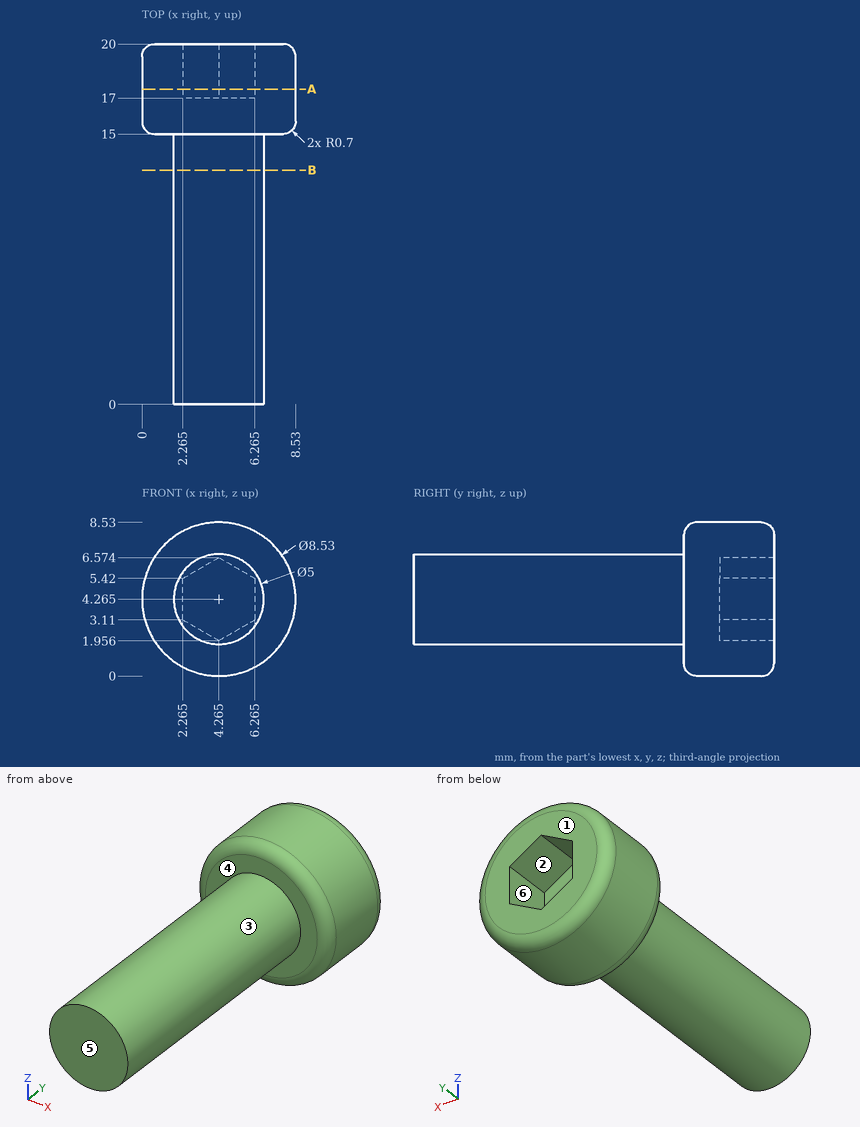
Design review of the part shown in the three views and the two pictorial views. Dimensions are in mm from the part's minimum x, y and z. A direction names the side the tool comes from. Round coordinates to 2 decimals unless told otherwise and drop trailing zeros. Loops run counter-clockwise (first coordinate to the right, second up) from the corner with the lowest first, then second, coordinate; pieces in that order, holes last. Notation, with made-up numbers: M -15.5,9 L 31.5,9 A27 ccw 31.5,26 Z; hole C -39.5,50 d2. An arc over 180 degrees is marked long. Put each result on its own line as item: value.
Q1. Mouldability with a two-part tool opening along X and no side actions: class the marked faces 1, 2 and 3 as released by +X, released by -X, zero draft, split by the parting line, or undercut.
Result set:
face 1: zero draft
face 2: undercut
face 3: split by the parting line
Q2. For pin 1 (4 mm diameter, centred on y = 12.5, z = 6.5, fed in from +X), flat-tipped, find the tip position at first contact; note if it passes through.
Result set:
pin 1: stops at x = 6.75
Q3. Consider section B-B, the plane y = 13. Give the boundary of the cut face in (x, z) (1 decimal).
Result set:
outline: C 4.3,4.3 d5
Q4. To check wall thickness, follow L1, parallel to Y at x = 2.5, z = 5.5; L2, parallel to Z at x = 0.5, y = 17 (1 decimal); L3, parallel to Y at x = 1.5, z = 5.5. State the ranges of each line that lie inside material, in increasing order.
Result set:
L1: y = 0 to 17
L2: z = 2.3 to 6.3
L3: y = 15 to 20
Q5. Consider section A-A, the plane y = 17.5. Give the boundary of the cut face in (x, z) (1 decimal).
Result set:
outline: C 4.3,4.3 d8.5; hole M 2.3,3.1 L 4.3,2 L 6.3,3.1 L 6.3,5.4 L 4.3,6.6 L 2.3,5.4 Z
Q6. Machinability: for the marked faces 4, 5 and 6, which of the approach directions +Z, -Z, +X, -X, +Y, -Y give a long, thin tool a straight path to every point of the face, cutting with its end or side? Answer none if there is none.
Result set:
face 4: -Y
face 5: +Z, -Z, +X, -X, -Y
face 6: +Y
